Input: part model. Units: mm. Frame: model coordinates. Face numbers are marked on the shaded views. A direction names the side the tool comes from. Round coordinates to 2 decimals unless told otherwise and drop trailing zeros. Loops run counter-clockwise (first coordinate to the right, second up) from the corner with the lowest first, then second, coordinate; pieces in that order, holes last. Notation, with made-up numbers: (5.5, -31) - (26.5, -31) arc R14 cw to (26.5, -7) - close; hole circle Ø6 at (-26.75, 6.25). An arc over 180 degrees is marked (long way). Write each question's results on one line, items separated by ' | '.
Autodesk Inventor part; units mm, degrees
ref_plane "Work Plane1" through (17.341, -12.884, 3.2549) normal (0, 0, -1) x (0, 1, 0)
ref_plane "YZ Plane" through (0, 0, 0) normal (1, 0, 0) x (0, 1, 0)
ref_plane "XZ Plane" through (0, 0, 0) normal (0, 1, 0) x (-1, 0, 0)
sketch "Sketch1" plane through (0, 0, 0) normal (0, 0, 1) x (1, 0, 0)
  circle A0 centre (0, -8) radius 12.065
  arc A1 (-7.912, -62.1223) -> (-4.7827, -62.4881) centre (0, -8) ccw
  arc A2 (-3.3911, -60.1215) -> (-4.7827, -62.4881) centre (5.3956, -66.8807) ccw
  arc A3 (3.3911, -60.1215) -> (-3.3911, -60.1215) centre (0, -62.6976) ccw
  arc A4 (4.7827, -62.4881) -> (3.3911, -60.1215) centre (-5.3956, -66.8807) ccw
  arc A5 (4.7827, -62.4881) -> (7.912, -62.1223) centre (0, -8) ccw
  arc A6 (8.7203, -59.4986) -> (7.912, -62.1223) centre (18.829, -64.0493) ccw
  arc A7 (15.3198, -57.9345) -> (8.7203, -59.4986) centre (12.6141, -61.2232) ccw
  arc A8 (17.2196, -59.9164) -> (15.3198, -57.9345) centre (8.3287, -66.5379) ccw
  arc A9 (17.2196, -59.9164) -> (20.1802, -58.8388) centre (0, -8) ccw
  arc A10 (20.3617, -56.0994) -> (20.1802, -58.8388) centre (31.2473, -58.1962) ccw
  arc A11 (26.4225, -53.0555) -> (20.3617, -56.0994) centre (24.5482, -56.8795) ccw
  arc A12 (28.7282, -54.5458) -> (26.4225, -53.0555) centre (21.6039, -63.0393) ccw
  arc A13 (28.7282, -54.5458) -> (31.3605, -52.8146) centre (0, -8) ccw
  arc A14 (30.9053, -50.1072) -> (31.3605, -52.8146) centre (41.9811, -49.637) ccw
  arc A15 (36.1008, -45.7476) -> (30.9053, -50.1072) centre (35.1589, -49.9008) ccw
  arc A16 (38.688, -46.666) -> (36.1008, -45.7476) centre (33.7145, -56.5735) ccw
  arc A17 (38.688, -46.666) -> (40.8501, -44.3744) centre (0, -8) ccw
  arc A18 (39.7828, -41.8449) -> (40.8501, -44.3744) centre (50.4517, -38.8332) ccw
  arc A19 (43.8329, -36.4047) -> (39.7828, -41.8449) centre (43.8742, -40.6631) ccw
  arc A20 (46.5622, -36.7017) -> (43.8329, -36.4047) centre (44.0076, -47.4891) ccw
  arc A21 (46.5622, -36.7017) -> (48.1375, -33.9732) centre (0, -8) ccw
  arc A22 (46.5156, -31.7581) -> (48.1375, -33.9732) centre (56.2023, -26.3671) ccw
  arc A23 (49.2019, -25.5305) -> (46.5156, -31.7581) centre (50.2242, -29.6646) ccw
  arc A24 (51.9262, -25.19) -> (49.2019, -25.5305) centre (51.9282, -36.2758) ccw
  arc A25 (51.9262, -25.19) -> (52.8298, -22.1718) centre (0, -8) ccw
  arc A26 (50.7408, -20.3904) -> (52.8298, -22.1718) centre (58.9232, -12.9109) ccw
  arc A27 (51.9185, -13.7112) -> (50.7408, -20.3904) centre (53.8666, -17.4981) ccw
  arc A28 (54.4908, -12.7517) -> (51.9185, -13.7112) centre (57.0493, -23.5382) ccw
  arc A29 (54.4908, -12.7517) -> (54.674, -9.6064) centre (0, -8) ccw
  arc A30 (52.2305, -8.3548) -> (54.674, -9.6064) centre (58.4674, 0.8101) ccw
  arc A31 (51.8361, -1.584) -> (52.2305, -8.3548) centre (54.605, -4.8196) ccw
  arc A32 (54.1178, -0.0572) -> (51.8361, -1.584) centre (59.0949, -9.9629) ccw
  arc A33 (54.1178, -0.0572) -> (53.5707, 3.0455) centre (0, -8) ccw
  arc A34 (50.9044, 3.6999) -> (53.5707, 3.0455) centre (54.8597, 14.0561) ccw
  arc A35 (48.9593, 10.1973) -> (50.9044, 3.6999) centre (52.3997, 7.6874) ccw
  arc A36 (50.8273, 12.2092) -> (48.9593, 10.1973) centre (57.9546, 3.7182) ccw
  arc A37 (50.8273, 12.2092) -> (49.5794, 15.1021) centre (0, -8) ccw
  arc A38 (46.8341, 15.1239) -> (49.5794, 15.1021) centre (48.2944, 26.1131) ccw
  arc A39 (43.443, 20.9975) -> (46.8341, 15.1239) centre (47.3695, 19.3488) ccw
  arc A40 (44.7967, 23.386) -> (43.443, 20.9975) centre (53.69, 16.7676) ccw
  arc A41 (44.7967, 23.386) -> (42.9153, 25.9131) centre (0, -8) ccw
  arc A42 (40.2389, 25.3013) -> (42.9153, 25.9131) centre (39.1256, 36.331) ccw
  arc A43 (35.5847, 30.2346) -> (40.2389, 25.3013) centre (39.7856, 29.5357) ccw
  arc A44 (36.3511, 32.8708) -> (35.5847, 30.2346) centre (46.531, 28.4818) ccw
  arc A45 (36.3511, 32.8708) -> (33.9376, 34.896) centre (0, -8) ccw
  arc A46 (31.4745, 33.6834) -> (33.9376, 34.896) centre (27.8475, 44.1591) ccw
  arc A47 (25.808, 37.4103) -> (31.4745, 33.6834) centre (30.0568, 37.6992) ccw
  arc A48 (25.9458, 40.1523) -> (25.808, 37.4103) centre (36.8635, 38.2292) ccw
  arc A49 (25.9458, 40.1523) -> (23.1303, 41.5662) centre (0, -8) ccw
  arc A50 (21.0132, 39.8183) -> (23.1303, 41.5662) centre (15.0682, 49.1752) ccw
  arc A51 (14.64, 42.138) -> (21.0132, 39.8183) centre (18.7077, 43.3989) ccw
  arc A52 (14.1417, 44.8378) -> (14.64, 42.138) centre (25.2086, 45.4844) ccw
  arc A53 (14.1417, 44.8378) -> (11.0761, 45.5644) centre (0, -8) ccw
  arc A54 (9.4191, 43.3754) -> (11.0761, 45.5644) centre (1.4765, 51.109) ccw
  arc A55 (2.6827, 44.1627) -> (9.4191, 43.3754) centre (6.35, 46.3277) ccw
  arc A56 (1.5753, 46.6749) -> (2.6827, 44.1627) centre (12.1948, 49.8562) ccw
  arc A57 (1.5753, 46.6749) -> (-1.5753, 46.6749) centre (0, -8) ccw
  arc A58 (-2.6827, 44.1627) -> (-1.5753, 46.6749) centre (-12.1948, 49.8562) ccw
  arc A59 (-9.4191, 43.3754) -> (-2.6827, 44.1627) centre (-6.35, 46.3277) ccw
  arc A60 (-11.0761, 45.5644) -> (-9.4191, 43.3754) centre (-1.4765, 51.109) ccw
  arc A61 (-11.0761, 45.5644) -> (-14.1417, 44.8378) centre (0, -8) ccw
  arc A62 (-14.64, 42.138) -> (-14.1417, 44.8378) centre (-25.2086, 45.4844) ccw
  arc A63 (-21.0132, 39.8183) -> (-14.64, 42.138) centre (-18.7077, 43.3989) ccw
  arc A64 (-23.1303, 41.5662) -> (-21.0132, 39.8183) centre (-15.0682, 49.1752) ccw
  arc A65 (-23.1303, 41.5662) -> (-25.9458, 40.1523) centre (0, -8) ccw
  arc A66 (-25.808, 37.4103) -> (-25.9458, 40.1523) centre (-36.8635, 38.2292) ccw
  arc A67 (-31.4745, 33.6834) -> (-25.808, 37.4103) centre (-30.0568, 37.6992) ccw
  arc A68 (-33.9376, 34.896) -> (-31.4745, 33.6834) centre (-27.8475, 44.1591) ccw
  arc A69 (-33.9376, 34.896) -> (-36.3511, 32.8708) centre (0, -8) ccw
  arc A70 (-35.5847, 30.2346) -> (-36.3511, 32.8708) centre (-46.531, 28.4818) ccw
  arc A71 (-40.2389, 25.3013) -> (-35.5847, 30.2346) centre (-39.7856, 29.5357) ccw
  arc A72 (-42.9153, 25.9131) -> (-40.2389, 25.3013) centre (-39.1256, 36.331) ccw
  arc A73 (-42.9153, 25.9131) -> (-44.7967, 23.386) centre (0, -8) ccw
  arc A74 (-43.443, 20.9975) -> (-44.7967, 23.386) centre (-53.69, 16.7676) ccw
  arc A75 (-46.8341, 15.1239) -> (-43.443, 20.9975) centre (-47.3695, 19.3488) ccw
  arc A76 (-49.5794, 15.1021) -> (-46.8341, 15.1239) centre (-48.2944, 26.1131) ccw
  arc A77 (-49.5794, 15.1021) -> (-50.8273, 12.2092) centre (0, -8) ccw
  arc A78 (-48.9593, 10.1973) -> (-50.8273, 12.2092) centre (-57.9546, 3.7182) ccw
  arc A79 (-50.9044, 3.6999) -> (-48.9593, 10.1973) centre (-52.3997, 7.6874) ccw
  arc A80 (-53.5707, 3.0455) -> (-50.9044, 3.6999) centre (-54.8597, 14.0561) ccw
  arc A81 (-53.5707, 3.0455) -> (-54.1178, -0.0572) centre (0, -8) ccw
  arc A82 (-51.8361, -1.584) -> (-54.1178, -0.0572) centre (-59.0949, -9.9629) ccw
  arc A83 (-52.2305, -8.3548) -> (-51.8361, -1.584) centre (-54.605, -4.8196) ccw
  arc A84 (-54.674, -9.6064) -> (-52.2305, -8.3548) centre (-58.4674, 0.8101) ccw
  arc A85 (-54.674, -9.6064) -> (-54.4908, -12.7517) centre (0, -8) ccw
  arc A86 (-51.9185, -13.7112) -> (-54.4908, -12.7517) centre (-57.0493, -23.5382) ccw
  arc A87 (-50.7408, -20.3904) -> (-51.9185, -13.7112) centre (-53.8666, -17.4981) ccw
  arc A88 (-52.8298, -22.1718) -> (-50.7408, -20.3904) centre (-58.9232, -12.9109) ccw
  arc A89 (-52.8298, -22.1718) -> (-51.9262, -25.19) centre (0, -8) ccw
  arc A90 (-49.2019, -25.5305) -> (-51.9262, -25.19) centre (-51.9282, -36.2758) ccw
  arc A91 (-46.5156, -31.7581) -> (-49.2019, -25.5305) centre (-50.2242, -29.6646) ccw
  arc A92 (-48.1375, -33.9732) -> (-46.5156, -31.7581) centre (-56.2023, -26.3671) ccw
  arc A93 (-48.1375, -33.9732) -> (-46.5622, -36.7017) centre (0, -8) ccw
  arc A94 (-43.8329, -36.4047) -> (-46.5622, -36.7017) centre (-44.0076, -47.4891) ccw
  arc A95 (-39.7828, -41.8449) -> (-43.8329, -36.4047) centre (-43.8742, -40.6631) ccw
  arc A96 (-40.8501, -44.3744) -> (-39.7828, -41.8449) centre (-50.4517, -38.8332) ccw
  arc A97 (-40.8501, -44.3744) -> (-38.688, -46.666) centre (0, -8) ccw
  arc A98 (-36.1008, -45.7476) -> (-38.688, -46.666) centre (-33.7145, -56.5735) ccw
  arc A99 (-30.9053, -50.1072) -> (-36.1008, -45.7476) centre (-35.1589, -49.9008) ccw
  arc A100 (-31.3605, -52.8146) -> (-30.9053, -50.1072) centre (-41.9811, -49.637) ccw
  arc A101 (-31.3605, -52.8146) -> (-28.7282, -54.5458) centre (0, -8) ccw
  arc A102 (-26.4225, -53.0555) -> (-28.7282, -54.5458) centre (-21.6039, -63.0393) ccw
  arc A103 (-20.3617, -56.0994) -> (-26.4225, -53.0555) centre (-24.5482, -56.8795) ccw
  arc A104 (-20.1802, -58.8388) -> (-20.3617, -56.0994) centre (-31.2473, -58.1962) ccw
  arc A105 (-20.1802, -58.8388) -> (-17.2196, -59.9164) centre (0, -8) ccw
  arc A106 (-15.3198, -57.9345) -> (-17.2196, -59.9164) centre (-8.3287, -66.5379) ccw
  arc A107 (-8.7203, -59.4986) -> (-15.3198, -57.9345) centre (-12.6141, -61.2232) ccw
  arc A108 (-7.912, -62.1223) -> (-8.7203, -59.4986) centre (-18.829, -64.0493) ccw
  circle A109 centre (0, -8) radius 31.75
  circle A110 centre (-22.225, -8) radius 2.3812
  circle A111 centre (0, 14.225) radius 2.3812
  circle A112 centre (0, -30.225) radius 2.3812
  circle A113 centre (22.225, -8) radius 2.3812
  point P0 (0, 0)
  dimension "d0" = 63.5
extrude "Extrusion1" add sketch "Sketch1" along normal blind 6.35 contours A109 | A110 | A111 | A112 | A113
sketch "Sketch2" plane through (0, -8, 6.35) normal (0, 0, 1) x (1, 0, 0)
  circle A0 centre (0, 0) radius 31.75
  circle A1 centre (0, 0) radius 12.065
  circle A2 centre (22.225, 0) radius 4.7625
  circle A3 centre (0, -22.225) radius 4.7625
  circle A4 centre (-22.225, 0) radius 4.7625
  circle A5 centre (0, 22.225) radius 1.27
  circle A6 centre (0, 22.225) radius 4.7625
  circle A7 centre (-22.225, 0) radius 1.27
  circle A8 centre (0, -22.225) radius 1.27
  circle A9 centre (22.225, 0) radius 1.27
  point P0 (0, 8)
  dimension "d3" = 9.525
  dimension "d4" = 9.525
  dimension "d5" = 9.525
  dimension "d6" = 9.525
ref_plane "Work Plane1" through (17.341, -12.884, 3.2549) normal (0, 0, -1) x (0, 1, 0)
extrude "Extrusion2" cut sketch "Sketch2" against normal through all contours A5 | A7 | A8 | A9
extrude "Extrusion3" cut sketch "Sketch2" against normal blind 3.175 contours A2 | A3 | A4 | A6
sketch "Sketch3" plane through (0, -8, 6.35) normal (0, 0, 1) x (1, 0, 0)
  circle A0 centre (22.225, 0) radius 4.7625
  circle A1 centre (0, -22.225) radius 4.7625
  circle A2 centre (-22.225, 0) radius 4.7625
  circle A3 centre (0, 22.225) radius 4.7625
  circle A4 centre (0, 0) radius 12.065
  circle A5 centre (22.225, 0) radius 9.525
  circle A6 centre (0, -22.225) radius 9.525
  circle A7 centre (-22.225, 0) radius 9.525
  circle A8 centre (0, 22.225) radius 9.525
  circle A9 centre (0, 0) radius 17.4625
  circle A10 centre (0, 0) radius 31.75
  arc A11 (20.9547, -9.4399) -> (9.4399, -20.9547) centre (19.5891, -19.5891) ccw
  arc A12 (9.4399, 20.9547) -> (20.9547, 9.4399) centre (19.5891, 19.5891) ccw
  arc A13 (-20.9547, 9.4399) -> (-9.4399, 20.9547) centre (-19.5891, 19.5891) ccw
  arc A14 (-9.4399, -20.9547) -> (-20.9547, -9.4399) centre (-19.5891, -19.5891) ccw
  point P0 (0, 8)
  point P1 (20.9547, 9.4399)
  point P2 (31.75, 0)
  point P3 (0, 31.75)
  point P4 (9.4399, 20.9547)
  point P5 (-9.4399, 20.9547)
  point P6 (-31.75, 0)
  point P7 (-20.9547, 9.4399)
  point P8 (-20.9547, -9.4399)
  point P9 (0, -31.75)
  point P10 (-9.4399, -20.9547)
  dimension "d13" = 360
extrude "Extrusion4" cut sketch "Sketch3" against normal through all contours A12 A8 A10 A5 | A5 A10 A6 A11 | A8 A13 A7 A10 | A10 A7 A14 A6
properties part number "drive sprocket flange socket"
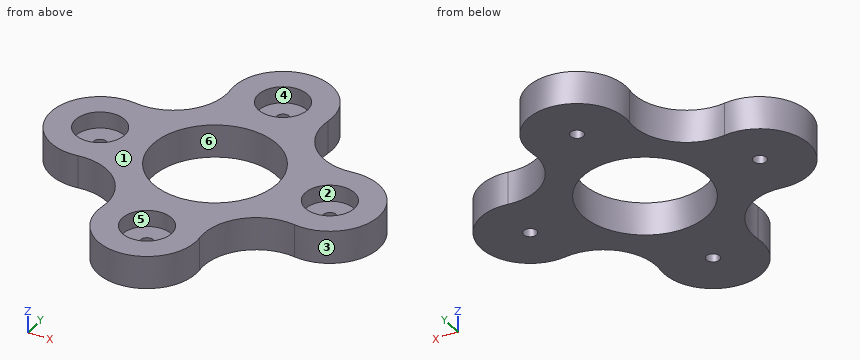
1. Mould query, pull axis Y, two halves, no side actions, for the marked faces 1, 2, 3 and 4. Classes: pulls with the +Y half, pulls with the -Y half, needs draft (parallel to the pull), parting line crosses it, or undercut.
Answer:
face 1: needs draft | face 2: undercut | face 3: parting line crosses it | face 4: undercut
2. Section query C-C, the plane x = -11. Output: boundary loops of the cut face in (y, z), plus the area to 3 significant figures.
Answer:
outline: (-22.01, 0) - (-12.96, 0) - (-12.96, 6.35) - (-22.01, 6.35) - close; (-3.04, 0) - (6.01, 0) - (6.01, 6.35) - (-3.04, 6.35) - close | area: 115 mm^2
3. Set-up query: the marked faces 5 and 6. Return all of +Z, -Z, +X, -X, +Y, -Y with unobstructed straight access to the full face (end or side cutting, diameter ignored); none if empty.
Answer:
face 5: +Z | face 6: +Z, -Z
4. Contact query for flat-ended pins moving along their axis: pin 1 (3 mm diameter, centred on x = 0.5, y = 12.5, fed in from +Z) (3 decimals); pin 2 (1.5 mm diameter, centred on x = -3, z = 5, fed in from +Y); pin 3 (1 mm diameter, centred on x = -12.5, z = 2.5, fed in from -Y). Output: stop coordinate, or through.
Answer:
pin 1: z = 3.175 | pin 2: y = 23.48 | pin 3: y = -20.71
5. Line query: line 1 (Y direction, x = 0, z = 1.75) (3 decimals); line 2 (Z direction, x = 4, y = -32) (3 decimals); line 3 (X direction, y = -16, z = 0.5). Output: solid intervals per line, ascending. Write a range as [from, to].
Answer:
line 1: [-39.75, -31.495], [-28.955, -20.065], [4.065, 12.955], [15.495, 23.75] | line 2: [0, 3.175] | line 3: [-27.39, -9.03], [9.03, 27.39]
6. Section query A-A, the plane y = -8. Count the separate pieces of the cut face and the enclosed holes in it, plus the area to 3 significant figures.
Answer:
separate pieces: 4 | enclosed holes: 0 | area: 173 mm^2
